The listing builds one solid part. Answer for the finished solid, in the listing's coordinates (mm). A direction names the side the tool comes from. Round coordinates to 2 decimals unless told otherwise and drop trailing zeros. Write each loop counter-clockwise with the first axis right and the second up, starting at its lowest first coordinate (ties: lowest second). Pieces come first, ordered by that corner, then holes. Notation, with made-up numbers: M -21.75,52 L -4.75,52 A14 ccw -4.75,63 Z; hole C 37.25,71.5 d3. An arc over 180 degrees is marked long. Answer as CSV lines item,"result". Start each with the question number.
from build123d import *

# Parameters (mm, degrees)
BOSS_EXTRUDE1_DEPTH = 4
BOSS_EXTRUDE3_START = 4
BOSS_EXTRUDE3_DEPTH = 1
CUT_EXTRUDE2_REACH  = 52.364
SKETCH5_R           = 1.25
SKETCH6_R           = 2.25
CUT_EXTRUDE3_DEPTH  = 2
SKETCH7_W           = 45
SKETCH7_H           = 2
CUT_EXTRUDE4_DEPTH  = 10


with BuildPart() as part:
    # Sketch1 → Boss-Extrude1 (new body)
    with BuildSketch(Plane(origin=(0, 0, 0), x_dir=(1, 0, 0), z_dir=(0, 1, 0))):
        Polygon((-35.5, 23), (-23, 35.5), (23, 35.5), (35.5, 23), (35.5, -23), (23, -35.5), (-23, -35.5), (-35.5, -23), align=None)
    extrude(amount=BOSS_EXTRUDE1_DEPTH)

    # Sketch3 → Boss-Extrude3 (add)
    with BuildSketch(Plane(origin=(0, 0, 0), x_dir=(1, 0, 0), z_dir=(0, 1, 0)).offset(BOSS_EXTRUDE3_START)):
        Polygon((-29.5, 20.514718626), (-20.514718626, 29.5), (20.514718626, 29.5), (29.5, 20.514718626), (29.5, -20.514718626), (20.514718626, -29.5), (-20.514718626, -29.5), (-29.5, -20.514718626), align=None)
    extrude(amount=BOSS_EXTRUDE3_DEPTH)

    # Sketch5 → Cut-Extrude2 (cut, up to next)
    with BuildSketch(Plane(origin=(0, 4, 0), x_dir=(1, 0, 0), z_dir=(0, 1, 0)), mode=Mode.PRIVATE) as cut_extrude2_sk1:
        with Locations(Location((32.5, 0, 0), (0, 0, 270))):
            Circle(SKETCH5_R)
    cut_extrude2_tool1 = extrude(cut_extrude2_sk1.sketch, amount=-CUT_EXTRUDE2_REACH, mode=Mode.PRIVATE) & part.part
    # Sketch5 → Cut-Extrude2 (cut, up to next)
    with BuildSketch(Plane(origin=(0, 4, 0), x_dir=(1, 0, 0), z_dir=(0, 1, 0)), mode=Mode.PRIVATE) as cut_extrude2_sk2:
        with Locations(Location((-32.5, 0, 0), (0, 0, 270))):
            Circle(SKETCH5_R)
    cut_extrude2_tool2 = extrude(cut_extrude2_sk2.sketch, amount=-CUT_EXTRUDE2_REACH, mode=Mode.PRIVATE) & part.part
    add(cut_extrude2_tool1.solids().sort_by_distance((32.5, 4, 0))[0], mode=Mode.SUBTRACT)
    add(cut_extrude2_tool2.solids().sort_by_distance((-32.5, 4, 0))[0], mode=Mode.SUBTRACT)

    # Sketch6 → Cut-Extrude3 (cut)
    with BuildSketch(Plane.XZ):
        with Locations(Location((32.5, 0, 0), (0, 0, 270))):
            Circle(SKETCH6_R)
        with Locations(Location((-32.5, 0, 0), (0, 0, 90))):
            Circle(SKETCH6_R)
    extrude(amount=-CUT_EXTRUDE3_DEPTH, mode=Mode.SUBTRACT)

    # Sketch7 → Cut-Extrude4 (cut)
    with BuildSketch(Plane.XZ):
        with Locations((0, 22.5)):
            Rectangle(SKETCH7_W, SKETCH7_H)
        with Locations((0, 17.5)):
            Rectangle(SKETCH7_W, SKETCH7_H)
        with Locations((0, 12.5)):
            Rectangle(SKETCH7_W, SKETCH7_H)
        with Locations((0, 7.5)):
            Rectangle(SKETCH7_W, SKETCH7_H)
        with Locations((0, 2.5)):
            Rectangle(SKETCH7_W, SKETCH7_H)
        with Locations((0, -2.5)):
            Rectangle(SKETCH7_W, SKETCH7_H)
        with Locations((0, -7.5)):
            Rectangle(SKETCH7_W, SKETCH7_H)
        with Locations((0, -12.5)):
            Rectangle(SKETCH7_W, SKETCH7_H)
        with Locations((0, -17.5)):
            Rectangle(SKETCH7_W, SKETCH7_H)
        with Locations((0, -22.5)):
            Rectangle(SKETCH7_W, SKETCH7_H)
    extrude(amount=-CUT_EXTRUDE4_DEPTH, mode=Mode.SUBTRACT)


solid = part.part
Q1. For faces 5 (the face through (0, 5, 0)), 6 (the face through (-22.5, 2, 7)), 7 (the face through (31.5, 2, -1)), determine the directions among +Z, -Z, +X, -X, +Y, -Y from which every point of the face is accessible in a straight line to the end or side of a thin tool.
Q2. The mould has two halves that part along X. Classify faces 1 (the face through (-29.2, 2, 29.3)), 2 (the face through (0, 0, 0)), 3 (the face through (29.2, 2, -29.3)), 4 (the face through (0, 2, 13.5)): +X half, -X half, draft (parallel to the pull), parting line (faces both ways), or undercut.
Q3. Find section C-C (x = -18.5). Count the separate pieces of the cut face and the enclosed holes in it, plus the area to 3 significant figures.
Q4. Find section A-A (z = 0). Determine the outline of the cut face in (x, y), plus the area to 3 significant figures.
Q5. Straight lines are drawn through the part: L1, parallel to X at y = 1.3, z = 0; L2, parallel to X at y = 3.4, z = 0; L3, parallel to X at y = 1.55, z = -23. For each, find the intervals that lie inside material, in ascending order.
Q6. Find section B-B (x = 32.5). Determine the outline of the cut face in (y, z), plus the area to 3 significant figures.
Q7. Each of these flat-tipped pins is pushed along its axis until it touches: P1, Ø1, axis at x = 13, z = -22.5, coming from the -Y side; P2, Ø4, axis at x = -32.5, z = 0, coming from the -Y side; P3, Ø0.5, axis at y = 4.5, z = -8.5, coming from the +X side. Where does it stop, or does it pass through?
Reported:
1,face 5,"+Z, -Z, +X, -X, +Y"
1,face 6,"+Y, -Y"
1,face 7,"-Y"
2,face 1,"-X half"
2,face 2,"draft"
2,face 3,"+X half"
2,face 4,"undercut"
3,separate pieces,"11"
3,enclosed holes,"0"
3,area,"243 mm2"
4,outline,"M -35.5,0 L -34.75,0 L -34.75,2 L -33.75,2 L -33.75,4 L -35.5,4 Z; M -31.25,2 L -30.25,2 L -30.25,0 L 30.25,0 L 30.25,2 L 31.25,2 L 31.25,4 L 29.5,4 L 29.5,5 L -29.5,5 L -29.5,4 L -31.25,4 Z; M 33.75,2 L 34.75,2 L 34.75,0 L 35.5,0 L 35.5,4 L 33.75,4 Z"
4,area,"315 mm2"
5,L1,"x = -35.5 to -34.75, -30.25 to 30.25, 34.75 to 35.5"
5,L2,"x = -35.5 to -33.75, -31.25 to 31.25, 33.75 to 35.5"
5,L3,"x = -35.5 to -22.5, 22.5 to 35.5"
6,outline,"M 0,-26 L 4,-26 L 4,-1.25 L 2,-1.25 L 2,-2.25 L 0,-2.25 Z; M 0,2.25 L 2,2.25 L 2,1.25 L 4,1.25 L 4,26 L 0,26 Z"
6,area,"194 mm2"
7,P1,"passes through"
7,P2,"stops at y = 2"
7,P3,"stops at x = 29.5"
